```python
from build123d import *

# Parameters (mm, degrees)
EXTRUDE_1_DEPTH              = 5
SKETCH_2_R                   = 6.25
EXTRUDE_2_DEPTH              = 3
HOLE_WIZARD_M4_1_D           = 3.3
HOLE_WIZARD_M4_1_DEPTH       = 5
HOLE_WIZARD_M4_1_TIP         = 0.991420021
EXTRUDE_3_DEPTH              = 5
EXTRUDE_4_DEPTH              = 5
HOLE_WIZARD_M3_1_D           = 3.4
HOLE_WIZARD_M3_1_CBORE_D     = 6.5
HOLE_WIZARD_M3_1_CBORE_DEPTH = 2
PATTERN_CIRCULAR_2_COUNT     = 3
PATTERN_CIRCULAR_3_COUNT     = 3
FILLET_1_R                   = 15


with BuildPart() as part:
    # 스케치1 → 보스-돌출1 (new body)
    with BuildSketch(Plane(origin=(0, 0, 0), x_dir=(1, 0, 0), z_dir=(0, 1, 0))):
        with BuildLine():
            Line((-15, 0), (-15, 60))
            ThreePointArc((-15, 60), (0, 75), (15, 60))
            Line((15, 60), (15, 0))
            ThreePointArc((15, 0), (0, -15), (-15, 0))
        make_face()
    extrude(amount=EXTRUDE_1_DEPTH)

    # 스케치2 → 보스-돌출2 (add)
    with BuildSketch(Plane(origin=(0, 5, 0), x_dir=(1, 0, 0), z_dir=(0, 1, 0))):
        with Locations(Location((0, 60, 0), (0, 0, 270))):
            Circle(SKETCH_2_R)
        with Locations(Location((0, 0, 0), (0, 0, 270))):
            Circle(SKETCH_2_R)
    extrude(amount=EXTRUDE_2_DEPTH)

    # M4 탭을 위한 탭 드릴1
    with Locations(Plane(origin=(0, 8, 0), x_dir=(1, 0, 0), z_dir=(0, 1, 0))):
        with Locations((0, 0), (0, 60)):
            Hole(HOLE_WIZARD_M4_1_D / 2, depth=HOLE_WIZARD_M4_1_DEPTH)
            with Locations((0, 0, -(HOLE_WIZARD_M4_1_DEPTH + HOLE_WIZARD_M4_1_TIP / 2))):  # 118° drill point
                Cone(0, HOLE_WIZARD_M4_1_D / 2, HOLE_WIZARD_M4_1_TIP, mode=Mode.SUBTRACT)

    # 스케치9 → 보스-돌출3 (add)
    with BuildSketch(Plane.XZ):
        with BuildLine():
            Line((-5.13030215, -14.095389312), (-33.321080773, -3.834785012))
            ThreePointArc((-33.321080773, -3.834785012), (-42.286167935, 15.39090645), (-23.060476474, 24.355993612))
            Line((-23.060476474, 24.355993612), (5.13030215, 14.095389312))
            ThreePointArc((5.13030215, 14.095389312), (14.095389312, -5.13030215), (-5.13030215, -14.095389312))
        make_face()
    extrude(amount=-EXTRUDE_3_DEPTH)

    # 스케치10 → 보스-돌출4 (add)
    with BuildSketch(Plane.XZ):
        with BuildLine():
            Line((-42.286167935, 15.39090645), (-32.025563636, 43.581685073))
            ThreePointArc((-32.025563636, 43.581685073), (-12.799872174, 52.546772235), (-3.834785012, 33.321080773))
            Line((-3.834785012, 33.321080773), (-14.095389312, 5.13030215))
            ThreePointArc((-14.095389312, 5.13030215), (-33.321080773, -3.834785012), (-42.286167935, 15.39090645))
        make_face()
    extrude(amount=-EXTRUDE_4_DEPTH)

    # M3 육각 소켓 머리 캡 나사용 카운터보어1 (through all)
    with Locations(Plane(origin=(0, 0, 0), x_dir=(-1, 0, 0), z_dir=(0, -1, 0))):
        with Locations((21.008355614, -29.994149336)):
            hole_wizard_m3_1 = CounterBoreHole(HOLE_WIZARD_M3_1_D / 2, HOLE_WIZARD_M3_1_CBORE_D / 2, HOLE_WIZARD_M3_1_CBORE_DEPTH)

    # 원형 패턴2: M3 육각 소켓 머리 캡 나사용 카운터보어1 ×3 about axis
    pattern_circular_2_axis = Axis((-17.930174324, 0, 38.451382923), (0, 1, 0))
    for i in range(1, PATTERN_CIRCULAR_2_COUNT):
        add(hole_wizard_m3_1.rotate(pattern_circular_2_axis, i * 360 / PATTERN_CIRCULAR_2_COUNT), mode=Mode.SUBTRACT)

    # 스케치18 → Ø5.0mm 맞춤핀 구멍1 (revolve, cut)
    with BuildSketch(Plane(origin=(-14.851993034, 5, 46.90861651), x_dir=(0, 0, 1), z_dir=(1, 0, 0))):
        Polygon((0, 0), (0, 4.002151548), (2.5, 2.5), (2.5, 0), align=None)
    f_5_0mm_1 = revolve(axis=Axis((-14.851993034, 11.35, 46.90861651), (0, -1, 0)), mode=Mode.SUBTRACT)

    # 원형 패턴3: Ø5.0mm 맞춤핀 구멍1 ×3 about axis
    pattern_circular_3_axis = Axis((-17.930174324, 0, 38.451382923), (0, 1, 0))
    for i in range(1, PATTERN_CIRCULAR_3_COUNT):
        add(f_5_0mm_1.rotate(pattern_circular_3_axis, i * 360 / PATTERN_CIRCULAR_3_COUNT), mode=Mode.SUBTRACT)

    # 필렛1
    fillet_1_edges = [part.edges().sort_by_distance(p)[0] for p in [
        (-8.965087162, 2.5, 19.225691462),
        (-15, 2.5, -10.503113073),
    ]]
    fillet(fillet_1_edges, radius=FILLET_1_R - 0.0001)  # a hair under: the kernel refuses the full size


solid = part.part
```
Check sheet for the modelled part. Datum: model origin and axes. Units: mm. A direction names the side the tool comes from. Round coordinates to 2 decimals unless told otherwise and drop trailing zeros. Order: outer loops, then holes, each group sorted by start corner. A loop starts at its lowest first (then second) coordinate and runs counter-clockwise, first axis right, second up. Notation, with made-up numbers: (80, 41.25) -> (104, 41.25) arc R17 ccw to (104, 54.25) -> close; hole circle Ø1 at (87.25, 52). An arc over 180 degrees is marked (long way). Use CSV: the item, a comma, the result in double quotes.
(1) Material ranges on line 1 along Z through (x, y) = (0.5, 6); line 2 along X through (y, z) = (3.25, 29.5); line 3 along Y through (x, z) = (-4, 18.5), recorded low to high. Write a range as from..to.
Worked out:
line 1,"-66.23..-61.57, -58.43..-53.77, -6.23..-1.57, 1.57..6.23"
line 2,"-37.15..-22.63, -19.38..-13.57, -10.72..-4.68"
line 3,"0..5"
(2) Cross-section at B-B (y = 6.5). Record the boundary of the cut face in (x, z), and give its area (3 significant figures).
Worked out:
outline,"circle Ø12.5 at (0, -60); circle Ø12.5 at (0, 0); hole circle Ø3.3 at (0, -60); hole circle Ø3.3 at (0, 0)"
area,"228 mm²"
(3) Draft check along X on faces 1 (the face through (-8.362, 0.986, 43.187)), 2 (the face through (-13.111, 2.465, 52.656)), 3 (the face through (15, 2, -30)), 4 (the face through (-1.3, 8, 1.3)). Enter one of: pulls with the +X half, pulls with the -X half, needs draft (parallel to the pull), parting line crosses it, or undercut.
Worked out:
face 1,"undercut"
face 2,"parting line crosses it"
face 3,"pulls with the +X half"
face 4,"needs draft"
(4) Cross-section at D-D (x = -38). Record the boundary of the cut face in (y, z).
Worked out:
outline,"(0, -1.09) -> (5, -1.09) -> (5, 27.17) -> (0, 27.17) -> close"
(5) Cross-section at C-C (x = 3). Record the boundary of the cut face in (y, z), and give its area (3 significant figures).
Worked out:
outline,"(0, -74.7) -> (5, -74.7) -> (5, -65.48) -> (8, -65.48) -> (8, -54.52) -> (5, -54.52) -> (5, -5.48) -> (8, -5.48) -> (8, 5.48) -> (5, 5.48) -> (5, 15.07) -> (0, 15.07) -> close"
area,"515 mm²"
(6) Tool access check on faces 5 (the face through (-18.61, 0.99, 27.8)), 6 (the face through (0.4, 5.5, -58.4)), 7 (the face through (-15, 2, -40)). Record the directions out of +Z, -Z, +X, -X, +Y, -Y that give a thin tool (end or side, any length) a straight path to the whole face; none if there is none.
Worked out:
face 5,"-Y"
face 6,"+Y"
face 7,"-Z, -X, +Y, -Y"
(7) Depth check by flat-ended pin: pin 1 (3 mm diameter, centred on x = -23.5, z = 46.5, fed in from -Y); pin 2 (2.5 mm diameter, centred on y = 2, z = -46.5, fed in from -X); pin 3 (5.5 mm diameter, centred on x = -9.07, z = 40.01, fed in from +Y). Enter the tip coordinate at first touch or a pass-through.
Worked out:
pin 1,"y = 2"
pin 2,"x = -15"
pin 3,"y = 5"
(8) Cross-section at A-A (z = -55). Record the boundary of the cut face in (x, y), and give its area (4 significant figures).
Worked out:
outline,"(-15, 0) -> (15, 0) -> (15, 5) -> (3.75, 5) -> (3.75, 8) -> (-3.75, 8) -> (-3.75, 5) -> (-15, 5) -> close"
area,"172.5 mm²"
